from build123d import *

# Parameters (mm, degrees)
F1_DEPTH = 27
F2_W     = 4.3404353922
F2_H     = 25
F3_DEPTH = 25


# Not quite as in the source:
# - a feature names something its author has since deleted; it is built from what else it names


with BuildPart() as f1:
    # F0 (on Top) → F1 (new body)
    with BuildSketch(Plane.XY):
        with BuildLine():
            Line((-9.8292995244, 17.7390783057), (-9.8292995244, 7.7390783057))
            Line((-9.8292995244, 7.7390783057), (-7.8292995244, 7.7390783057))
            Line((-7.8292995244, 7.7390783057), (-7.8292995244, 17.7390783057))
            ThreePointArc((-7.8292995244, 17.7390783057), (-8.8292995244, 23.5675054304), (-9.8292995244, 17.7390783057))
        make_face()
    extrude(amount=F1_DEPTH)

    # F2 (on Right) → F3 (cut)
    with BuildSketch(Plane.YZ):
        with Locations((19.9092960018, 13.5)):
            Rectangle(F2_W, F2_H)
    extrude(amount=-F3_DEPTH, mode=Mode.SUBTRACT)


solid = f1.part
The model under review builds one solid part; all positions refer to its coordinate system, in mm. A direction names the side the tool comes from. Coordinates: 2 decimals unless noted, no trailing zeros. Write each loop counter-clockwise with the first axis right and the second up, starting at its lowest first coordinate (ties: lowest second). Pieces come first, ordered by that corner, then holes. Notation, with made-up numbers: (83, -8) - (140, -8) arc R22 ccw to (140, 24) - close; hole circle Ø11 at (42, -29). An arc over 180 degrees is marked (long way). Answer as CSV lines item,"result".
(1) For line 1 along Z through (x, y) = (-8.95, 19.5); line 2 along Y through (x, z) = (-8.8, 21.75); line 3 along X through (y, z) = (14.25, 16), list the stretches that pass through material, from the lowest coordinate up. Write a range as [from, to].
Data:
line 1,"z = [0, 1], [26, 27]"
line 2,"y = [7.74, 17.74], [22.08, 23.57]"
line 3,"x = [-9.83, -7.83]"
(2) We need section C-C (x = -8.8). Give the boundary of the cut face in (y, z), plus the area to 3 significant figures.
Data:
outline,"(7.74, 0) - (23.57, 0) - (23.57, 27) - (7.74, 27) - close; hole (17.74, 1) - (22.08, 1) - (22.08, 26) - (17.74, 26) - close"
area,"319 mm2"
(3) Tool access review of faces 1 (the flat face through (-9, 7.739, 13)), 2 (the flat face through (-7.829, 13, 13)), 3 (the flat face through (-9, 20, 1)): name each direction out of +Z, -Z, +X, -X, +Y, -Y from which nothing blocks a thin tool from reaching the whole face with its end or side.
Data:
face 1,"+Z, -Z, +X, -X, -Y"
face 2,"+Z, -Z, +X, -Y"
face 3,"+X, -X"
(4) We need section D-D (x = -6.65). Give the boundary of the cut face in (y, z), plus the area to 3 significant figures.
Data:
outline,"(18.51, 0) - (22.63, 0) - (22.63, 27) - (18.51, 27) - (18.51, 26) - (22.08, 26) - (22.08, 1) - (18.51, 1) - close"
area,"22.0 mm2"
(5) We need section A-A (z = 19). Give the boundary of the cut face in (x, y).
Data:
outline,"(-11.42, 22.08) - (-6.24, 22.08) arc R3 ccw to start; (-9.83, 7.74) - (-7.83, 7.74) - (-7.83, 17.74) - (-9.83, 17.74) - close"
(6) Mouldability with a two-part tool opening along Z and no side actions: class faces 4 (the flat face through (-9.829, 13, 13)), 5 (the flat face through (-9, 18, 27)), 6 (the flat face through (-9, 20, 26)) as pulls with the +Z half, pulls with the -Z half, needs draft (parallel to the pull), parting line crosses it, or undercut.
Data:
face 4,"needs draft"
face 5,"pulls with the +Z half"
face 6,"undercut"
(7) We need section B-B (y = 18.75). Give the boundary of the cut face in (x, z), plus the area to 3 significant figures.
Data:
outline,"(-11.22, 0) - (-6.44, 0) - (-6.44, 1) - (-11.22, 1) - close; (-11.22, 26) - (-6.44, 26) - (-6.44, 27) - (-11.22, 27) - close"
area,"9.55 mm2"
(8) Clearance check with flat-ended pins moving along their axes: pin 1 Ø1 at (x, y) = (-7.5, 9.5) entering from -Z; pin 2 Ø3 at (y, z) = (14, 8) entering from -X; pin 3 Ø3 at (y, z) = (21, 5.5) entering from -X. State where each tip first meets the part, or that it passes through.
Data:
pin 1,"stops at z = 0"
pin 2,"stops at x = -9.83"
pin 3,"stops at x = -11.42"
